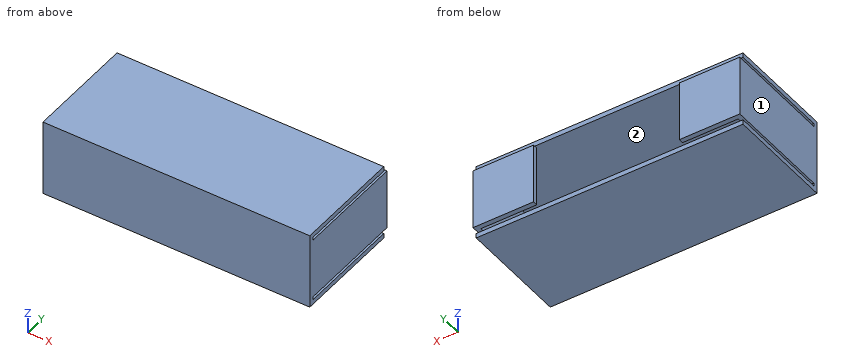
```python
from build123d import *

# Parameters (mm, degrees)
SKETCH1_W           = 56
SKETCH1_H           = 16
BOSS_EXTRUDE1_DEPTH = 1
BOSS_EXTRUDE2_DEPTH = 22
SKETCH3_W           = 1
SKETCH3_H           = 12.73
BOSS_EXTRUDE3_DEPTH = 22
SKETCH4_W           = 12.7
SKETCH4_H           = 12.73
BOSS_EXTRUDE4_DEPTH = 1


with BuildPart() as part:
    # Sketch1 → Boss-Extrude1 (new body)
    with BuildSketch(Plane(origin=(0, 0, 0), x_dir=(1, 0, 0), z_dir=(0, 1, 0))):
        Rectangle(SKETCH1_W, SKETCH1_H)
    extrude(amount=BOSS_EXTRUDE1_DEPTH)

    # Sketch2 → Boss-Extrude2 (add)
    with BuildSketch(Plane(origin=(0, 1, 0), x_dir=(1, 0, 0), z_dir=(0, 1, 0))):
        Polygon((28, -7), (27, -7), (-27, -7), (-28, -7), (-28, -8), (28, -8), align=None)
        Polygon((-27, 7), (27, 7), (28, 7), (28, 8), (-28, 8), (-28, 7), align=None)
    extrude(amount=BOSS_EXTRUDE2_DEPTH)

    # Sketch3 → Boss-Extrude3 (add)
    with BuildSketch(Plane(origin=(0, 1, 0), x_dir=(1, 0, 0), z_dir=(0, 1, 0))):
        with Locations((27.5, 0)):
            Rectangle(SKETCH3_W, SKETCH3_H)
        with Locations((-27.5, 0)):
            Rectangle(SKETCH3_W, SKETCH3_H)
    extrude(amount=BOSS_EXTRUDE3_DEPTH)

    # Sketch4 → Boss-Extrude4 (add)
    with BuildSketch(Plane(origin=(0, 23, 0), x_dir=(1, 0, 0), z_dir=(0, 1, 0))):
        with Locations((-21.65, 0)):
            Rectangle(SKETCH4_W, SKETCH4_H)
        with Locations((21.65, 0)):
            Rectangle(SKETCH4_W, SKETCH4_H)
    extrude(amount=BOSS_EXTRUDE4_DEPTH)


solid = part.part
```
Geometry check sheet. Reference: the model listing, model coordinates, mm. Face numbers are marked on the shaded views. A direction names the side the tool comes from. Coordinates: 2 decimals unless noted, no trailing zeros. Order: outer loops, then holes, each group sorted by start corner. A loop starts at its lowest first (then second) coordinate and runs counter-clockwise, first axis right, second up. Notation, with made-up numbers: M -32,-30.5 L -14,-30.5 A21 cw -14,0.5 Z; hole C 89,-6 d7. An arc over 180 degrees is marked long. Answer as a JSON object with one key per item and string values.
Q1. Cross-section at C-C on z = -3. Record the cut outline in (x, y).
Results are:
{"outline": "M -28,0 L 28,0 L 28,24 L 15.3,24 L 15.3,23 L 27,23 L 27,1 L -27,1 L -27,23 L -15.3,23 L -15.3,24 L -28,24 Z"}
Q2. Tool access check on the marked faces 1 and 2. Record the directions out of +Z, -Z, +X, -X, +Y, -Y that give a thin tool (end or side, any length) a straight path to the whole face; none if there is none.
Results are:
{"face 1": "+Z, -Z, -X, +Y, -Y", "face 2": "+X, -X, +Y"}
Q3. Scan lines: line 1 (Z direction, x = -1.5, y = 10.75); line 2 (X direction, y = 3.5, z = -5.25); line 3 (Y direction, x = -26, z = 5.25). Record each from-to range of solid material in increasing order.
Results are:
{"line 1": "z = -8 to -7, 7 to 8", "line 2": "x = -28 to -27, 27 to 28", "line 3": "y = 0 to 1, 23 to 24"}
Q4. Cross-section at B-B on x = 22. Record the cut outline in (y, z) (3 decimals), and give its area (3 significant figures).
Results are:
{"outline": "M 0,-8 L 23,-8 L 23,-7 L 1,-7 L 1,7 L 23,7 L 23,8 L 0,8 Z; M 23,-6.365 L 24,-6.365 L 24,6.365 L 23,6.365 Z", "area": "72.7 mm²"}
Q5. Cross-section at D-D on x = -10.5. Record the cut outline in (y, z).
Results are:
{"outline": "M 0,-8 L 23,-8 L 23,-7 L 1,-7 L 1,7 L 23,7 L 23,8 L 0,8 Z"}
Q6. Depth check by flat-ended pin: pin 1 Ø5 at (x, z) = (-3.5, -2.5) entering from +Y. Enter the tip coordinate at first touch or a pass-through.
Results are:
{"pin 1": "stops at y = 1"}
Q7. Cross-section at A-A on y = 8. Record the cut outline in (x, z) (3 decimals), and give its area (3 significant figures).
Results are:
{"outline": "M -28,-8 L 28,-8 L 28,-7 L -28,-7 Z; M -28,-6.365 L -27,-6.365 L -27,6.365 L -28,6.365 Z; M -28,7 L 28,7 L 28,8 L -28,8 Z; M 27,-6.365 L 28,-6.365 L 28,6.365 L 27,6.365 Z", "area": "137 mm²"}
